The drawing under review shows one solid part. Ordinate dimensions are in mm from its lowest x, y, z. Give positions to 0.01 mm unless a question says otherwise; leave off trailing zeros. Order: outer loops, then holes, each group sorted by start corner. A loop starts at its lowest first (then second) coordinate and runs counter-clockwise, first axis right, second up. Notation, with made-up numbers: (37, 54.25) -> (51, 54.25) arc R10 cw to (51, 58.25) -> close; hole circle Ø7 at (-11, 7.5). An arc over 180 degrees is marked (long way). Use a Markdown table: item, result. Add a question column.
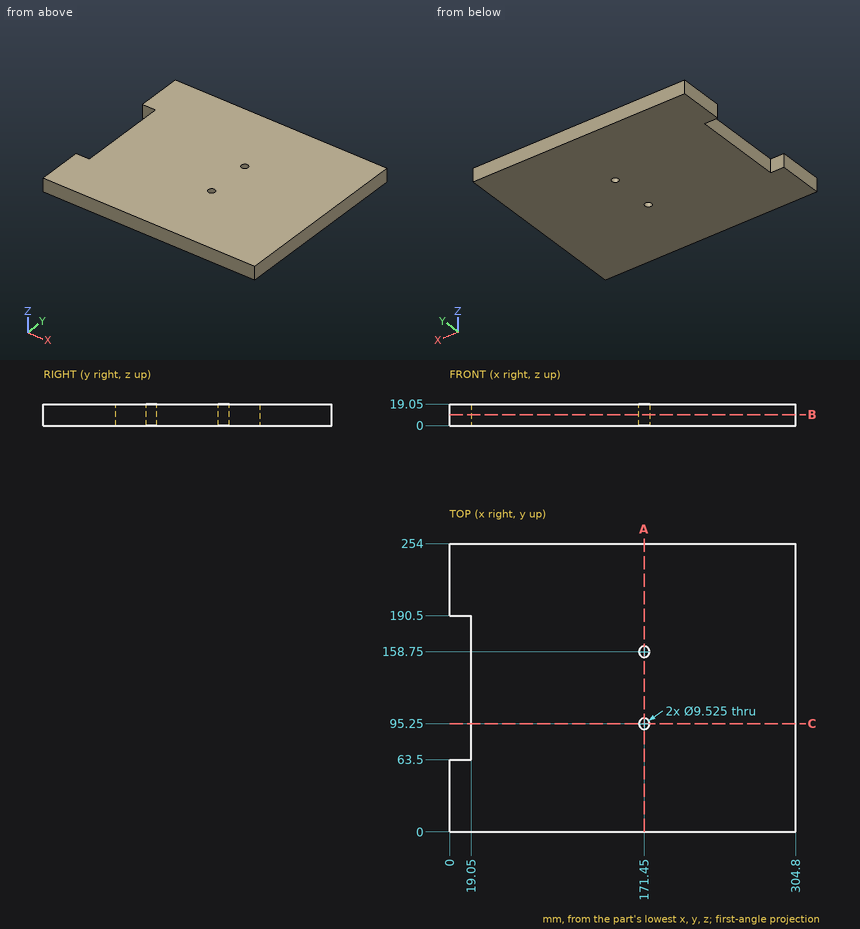
1) Add section C-C (y = 95.25). Give the boundary of the cut face in (x, z).
2) Add section A-A (x = 171.45). Give the boundary of the cut face in (y, z), then the cut area to 3 significant figures.
3) Add section B-B (z = 9.75). Give the number of separate pieces and of enclosed holes in the cut face, then the cut area to 3 significant figures.
4) Insertion check: pin 1 (1.5 mm diameter, centred on y = 57, z = 3, fed in from -X). The pin has a flat end and moves straight along its axis. Give the tip position at first contact, or say it passes through.
5) For L1, parallel to Y at x = 171.45, z = 7.5; L2, parallel to Y at x = 173, z = 4.5; L3, parallel to X at y = 121, z = 14, list the stretches that pass through material, from the lowest coordinate up. Write a range as [from, to].
Worked answers:
| question | item | result |
|---|---|---|
| 1 | outline | (19.05, 0) -> (166.69, 0) -> (166.69, 19.05) -> (19.05, 19.05) -> close; (176.21, 0) -> (304.8, 0) -> (304.8, 19.05) -> (176.21, 19.05) -> close |
| 2 | outline | (0, 0) -> (90.49, 0) -> (90.49, 19.05) -> (0, 19.05) -> close; (100.01, 0) -> (153.99, 0) -> (153.99, 19.05) -> (100.01, 19.05) -> close; (163.51, 0) -> (254, 0) -> (254, 19.05) -> (163.51, 19.05) -> close |
| 2 | area | 4,480 mm^2 |
| 3 | separate pieces | 1 |
| 3 | enclosed holes | 2 |
| 3 | area | 74,900 mm^2 |
| 4 | pin 1 | x = 0 |
| 5 | L1 | [0, 90.49], [100.01, 153.99], [163.51, 254] |
| 5 | L2 | [0, 90.75], [99.75, 154.25], [163.25, 254] |
| 5 | L3 | [19.05, 304.8] |
